Can you work these out from the model? Positions are in its coordinate system, mm. A direction names the side the tool comes from. Give positions to 0.01 mm unless a question says otherwise; leave off trailing zeros. Loops run counter-clockwise (first coordinate to the right, second up) from the corner with the lowest first, then second, coordinate; pieces in that order, holes last.
from build123d import *

# Parameters (mm, degrees)
F0_R     = 12.5
F0_R_2   = 2.5
F1_DEPTH = 6
F0_R_3   = 22
F2_DEPTH = 10


with BuildPart() as f1:
    # F0 (on Front) → F1 (new body)
    with BuildSketch(Plane.XZ):
        Circle(F0_R)
        Circle(F0_R_2, mode=Mode.SUBTRACT)
    extrude(amount=F1_DEPTH)

    # F0 (on Front) → F2 (join)
    with BuildSketch(Plane.XZ):
        Circle(F0_R_3)
        Circle(F0_R, mode=Mode.SUBTRACT)
        Circle(F0_R)
        Circle(F0_R_2, mode=Mode.SUBTRACT)
    extrude(amount=-F2_DEPTH)


solid = f1.part
(1) Which directions (+Z, -Z, +X, -X, +Y, -Y) give clear straight access to the entire face, cutting with the end or side of a thin tool? Please do faces 1 (the flat face through (9, 0, -9)), 2 (the cylindrical face through (-4.769, 4.93, -21.477)).
Returned:
face 1: -Y
face 2: +Y, -Y
(2) Suppose I cut it at A-A on x = 0. List the corners of the cut face in (y, z) for me, plus the area to 3 significant figures.
Returned:
outline: (-6, -12.5) - (0, -12.5) - (0, -22) - (10, -22) - (10, -2.5) - (-6, -2.5) - close; (-6, 2.5) - (10, 2.5) - (10, 22) - (0, 22) - (0, 12.5) - (-6, 12.5) - close
area: 510 mm2
(3) Will these pins go through, and if not, where does the flat tip stop? P1, Ø1, axis at y = -3.5, z = -9, coming from the -X side; P2, Ø5, axis at x = -1.5, y = -3.5, coming from the +Z side; P3, Ø2, axis at x = -6.5, z = 15, coming from the -Y side.
Returned:
P1: stops at x = -9.17
P2: stops at z = 12.5
P3: stops at y = 0
(4) Suppose I cut it at C-C on y = -3.5. List the corners of the cut face in (x, z) for me.
Returned:
outline: circle Ø25 at (0, 0); hole circle Ø5 at (0, 0)
(5) Suppose I cut it at B-B on z = 0. List the corners of the cut face in (x, y) for me.
Returned:
outline: (-22, 0) - (-12.5, 0) - (-12.5, -6) - (-2.5, -6) - (-2.5, 10) - (-22, 10) - close; (2.5, -6) - (12.5, -6) - (12.5, 0) - (22, 0) - (22, 10) - (2.5, 10) - close
(6) Please list where these lines run through material, in increasing order: probe 1 along Z at (x, y) = (0, -4.3); probe 2 along Y at (x, z) = (16, 11); probe 3 along X at (y, z) = (-4.25, 1.5).
Returned:
probe 1: z = -12.5 to -2.5, 2.5 to 12.5
probe 2: y = 0 to 10
probe 3: x = -12.41 to -2, 2 to 12.41
(7) Suppose I cut it at D-D on z = 7. List the corners of the cut face in (x, y) for me.
Returned:
outline: (-20.86, 0) - (-10.36, 0) - (-10.36, -6) - (10.36, -6) - (10.36, 0) - (20.86, 0) - (20.86, 10) - (-20.86, 10) - close
